```python
from build123d import *

# Parameters (mm, degrees)
BOSS_EXTRUDE1_START             = -411.784875
SKETCH3_R                       = 24.13
BOSS_EXTRUDE1_DEPTH             = 823.56975
CHAMFER1_SIZE                   = 0.254
BOSS_EXTRUDE3_REACH             = 833.382
SKETCH6_R                       = 24.13
SKETCH6_R_2                     = 22.352
BOSS_EXTRUDE3_DIRECTION_2_REACH = 833.382
BOSS_EXTRUDE2_DEPTH             = 431.8
BOSS_EXTRUDE2_DEPTH_BACK        = 431.8
LPATTERN1_COUNT                 = 2
LPATTERN1_PITCH                 = 33.02
BOSS_EXTRUDE4_DEPTH             = 475
BOSS_EXTRUDE5_DEPTH             = 475


with BuildPart() as part:
    # Sketch2 → Revolve1 (revolve)
    with BuildSketch(Plane.XY, mode=Mode.PRIVATE) as revolve1_sk:
        Polygon((-417.5125, 0), (-417.5125, 11.1125), (-418.896875, 11.1125), (-418.896875, 15.712927565), (-413.562875, 15.712927565), (-413.562875, 20.574), (-418.896875, 20.574), (-418.896875, 24.13), (-417.118875, 24.13), (-417.118875, 22.352), (-411.784875, 22.352), (-411.784875, 0), align=None)
    revolve(revolve1_sk.sketch.rotate(Axis((-417.5125, 0, 0), (1, 0, 0)), 180), axis=Axis((-417.5125, 0, 0), (1, 0, 0)))


with BuildPart() as body_2:
    # Mirror2: mirrored copy
    add(part.part.mirror(Plane(origin=(0, 0, 0), x_dir=(0, 0, 1), z_dir=(1, 0, 0))))


with BuildPart() as part_1:
    add(part.part)

    add(body_2.part)  # Boss-Extrude1 merges body 2
    # Sketch3 → Boss-Extrude1 (add)
    with BuildSketch(Plane(origin=(0, 0, 0), x_dir=(0, 0, -1), z_dir=(1, 0, 0)).offset(BOSS_EXTRUDE1_START)):
        with Locations(Location((0, 0, 0), (0, 0, 270))):
            Circle(SKETCH3_R)
    extrude(amount=BOSS_EXTRUDE1_DEPTH)

    # Chamfer1
    chamfer1_edges = [part_1.edges().sort_by_distance(p)[0] for p in [
        (417.118875, 24.13, 0),
        (-417.118875, 24.13, 0),
    ]]
    chamfer(chamfer1_edges, length=CHAMFER1_SIZE)

    # Boss-Extrude3: up to this face of the body (flat: up to its plane)
    boss_extrude3_end = Plane(part_1.part.faces().sort_by_distance((-417.118875, 23.20068474, 0))[0])
    # Sketch6 → Boss-Extrude3 (add, up to the picked face)
    with BuildSketch(Plane.ZY.offset(411.784875), mode=Mode.PRIVATE) as boss_extrude3_sk1:
        with Locations(Location((0, 0, 0), (0, 0, 270))):
            Circle(SKETCH6_R)
        Circle(SKETCH6_R_2, mode=Mode.SUBTRACT)
    boss_extrude3_tool1 = split(extrude(boss_extrude3_sk1.sketch, amount=BOSS_EXTRUDE3_REACH, mode=Mode.PRIVATE), bisect_by=boss_extrude3_end, keep=Keep.BOTH, mode=Mode.PRIVATE)
    add(boss_extrude3_tool1.solids().sort_by(Axis((-411.784875, 23.447501, 0), (-1, 0, 0)))[0])

    # Boss-Extrude3 direction 2: up to this face of the body (flat: up to its plane)
    boss_extrude3_direction_2_end = Plane(part_1.part.faces().sort_by_distance((417.118875, 23.20068474, 0))[0])
    # Sketch6 → Boss-Extrude3 direction 2 (add, up to the picked face)
    with BuildSketch(Plane.ZY.offset(411.784875), mode=Mode.PRIVATE) as boss_extrude3_direction_2_sk1:
        with Locations(Location((0, 0, 0), (0, 0, 270))):
            Circle(SKETCH6_R)
        Circle(SKETCH6_R_2, mode=Mode.SUBTRACT)
    boss_extrude3_direction_2_tool1 = split(extrude(boss_extrude3_direction_2_sk1.sketch, amount=-BOSS_EXTRUDE3_DIRECTION_2_REACH, mode=Mode.PRIVATE), bisect_by=boss_extrude3_direction_2_end, keep=Keep.BOTH, mode=Mode.PRIVATE)
    add(boss_extrude3_direction_2_tool1.solids().sort_by(Axis((-411.784875, 23.447501, 0), (1, 0, 0)))[0])

    # Sketch4 → Boss-Extrude2 (add, two sides: drawn at the far end of the back side and taken through both)
    with BuildSketch(Plane(origin=(0, 0, 0), x_dir=(0, 0, -1), z_dir=(1, 0, 0)).offset(-BOSS_EXTRUDE2_DEPTH_BACK)):
        Polygon((0, 6.415804866), (-5.55625, 3.207902433), (-5.55625, -3.207902433), (0, -6.415804866), (5.55625, -3.207902433), (5.55625, 3.207902433), align=None)
    extrude(amount=BOSS_EXTRUDE2_DEPTH + BOSS_EXTRUDE2_DEPTH_BACK)

    # Sketch5 → Cut-Revolve1 (revolve, cut)
    with BuildSketch(Plane.XY, mode=Mode.PRIVATE) as cut_revolve1_sk:
        with BuildLine():
            Line((-357.18115, 24.8874), (-357.18115, 25.5224))
            Line((-357.18115, 25.5224), (-350.84385, 25.5224))
            Line((-350.84385, 25.5224), (-350.84385, 24.8874))
            ThreePointArc((-350.84385, 24.8874), (-351.40062588, 24.65677588), (-351.63125, 24.1))
            ThreePointArc((-351.63125, 24.1), (-354.0125, 21.71875), (-356.39375, 24.1))
            ThreePointArc((-356.39375, 24.1), (-356.62437412, 24.65677588), (-357.18115, 24.8874))
        make_face()
    cut_revolve1 = revolve(cut_revolve1_sk.sketch.rotate(Axis((-431.8, 0, 0), (1, 0, 0)), 180), axis=Axis((-431.8, 0, 0), (1, 0, 0)), mode=Mode.SUBTRACT)

    # LPattern1: Cut-Revolve1 ×2
    with Locations(*[(i * LPATTERN1_PITCH, 0, 0) for i in range(1, LPATTERN1_COUNT)]):
        add(cut_revolve1, mode=Mode.SUBTRACT)

    # Sketch4<3> → Boss-Extrude4 (add)
    with BuildSketch(Plane(origin=(0, 0, 0), x_dir=(0, 0, -1), z_dir=(1, 0, 0))):
        Polygon((0, 6.415804866), (-5.55625, 3.207902433), (-5.55625, -3.207902433), (0, -6.415804866), (5.55625, -3.207902433), (5.55625, 3.207902433), align=None)
    extrude(amount=BOSS_EXTRUDE4_DEPTH)

    # Sketch4<4> → Boss-Extrude5 (add)
    with BuildSketch(Plane(origin=(0, 0, 0), x_dir=(0, 0, -1), z_dir=(1, 0, 0))):
        Polygon((0, 6.415804866), (-5.55625, 3.207902433), (-5.55625, -3.207902433), (0, -6.415804866), (5.55625, -3.207902433), (5.55625, 3.207902433), align=None)
    extrude(amount=-BOSS_EXTRUDE5_DEPTH)


solid = part_1.part
```
Read the model definition and answer for the solid it produces. Units are mm, in the model's axes. A direction names the side the tool comes from. Give positions to 0.01 mm unless a question says otherwise; leave off trailing zeros. Loops run counter-clockwise (first coordinate to the right, second up) from the corner with the lowest first, then second, coordinate; pieces in that order, holes last.
Item 1: The mould has two halves that part along Y. Classify faces 4 (the flat face through (-417.512, -5, -3)), 5 (the cylindrical face through (54.404, -23.016, 7.248)), 6 (the flat face through (418.897, -11, 3)): released by +Y, released by -Y, zero draft, split by the parting line, or undercut.
Item 2: The part is cut by section A-A (x = -136). Write down the section's boundary in (y, z), and give its area (3 significant figures).
Item 3: Find the intervals of material crossed by line 1 along X through (y, z) = (21.5, -5); line 2 along X through (y, z) = (-17.5, 1); line 3 along Z through (x, y) = (-206, 3), in increasing order.
Item 4: For faces 1 (the cylindrical face through (418.124, -23.016, -7.248)), 2 (the cylindrical face through (416.193, -8.447, -13.249)), 3 (the cylindrical face through (-416.193, -8.447, -13.249)), determine the directions among +Z, -Z, +X, -X, +Y, -Y from which every point of the face is accessible in a straight line to the end or side of a thin tool.
Item 5: Each of these flat-tipped pins is pushed along its axis until it touches: pin 1 Ø1.5 at (x, z) = (171, -13) entering from -Y; pin 2 Ø5 at (x, y) = (440, -1) entering from +Z; pin 3 Ø1.5 at (x, y) = (-191, -9.5) entering from -Z. Where does it stop, or does it pass through?
Taken from the geometry:
1. face 4: undercut
1. face 5: split by the parting line
1. face 6: zero draft
2. outline: circle Ø48.26 at (0, 0)
2. area: 1,830 mm2
3. line 1: x = -418.9 to -355.26, -352.76 to -322.24, -319.74 to 418.9
3. line 2: x = -413.56 to 413.56
3. line 3: z = -23.94 to 23.94
4. face 1: +X, -X
4. face 2: +X
4. face 3: -X
5. pin 1: stops at y = -20.79
5. pin 2: stops at z = 5.56
5. pin 3: stops at z = -22.49
